Check sheet for the drawn part. Datum: minimum x, y, z corner. Units: mm. Coordinates: 2 decimals unless noted, no trailing zeros. Order: outer loops, then holes, each group sorted by start corner. A loop starts at its lowest first (then second) coordinate and runs counter-clockwise, first axis right, second up.
1. Cross-section at B-B (y = 23). Enter the section's corners in (x, z) (3 decimals).
2. Cross-section at A-A (z = 94). Enter the section's corners in (x, y) (3 decimals).
3. Gauge pin test, flat ends, axial feed: pin 1 Ø1.5 at (x, y) = (13, 133) entering from +Z; pin 2 Ø1.5 at (x, y) = (12, 131) entering from -Z; pin 3 Ø2.5 at (x, z) = (14, 68.5) entering from +Y. Record the tip position at first contact, or that the pin passes through.
4. Thickness scan on line 1 (Z direction, x = 14.75, y = 26); line 2 (X direction, y = 126, z = 55.5) (3 decimals); line 3 (Y direction, x = 15.25, z = 84.5). Record the ranges inside material, lowest first.
5. Cross-section at C-C (x = 6.35). Enter the section's corners in (y, z).
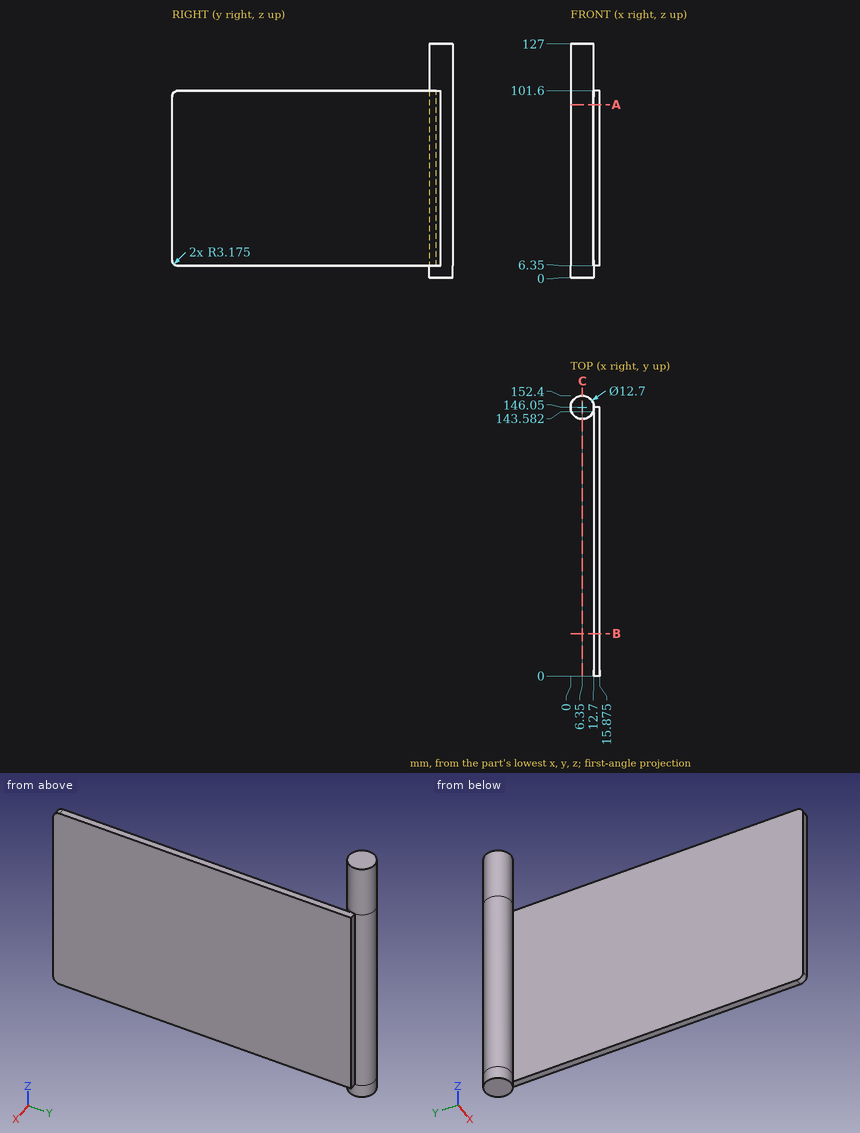
Data:
1. outline: (12.7, 6.35) - (15.875, 6.35) - (15.875, 101.6) - (12.7, 101.6) - close
2. outline: (12.201, 143.582) - (12.7, 143.582) - (12.7, 0) - (15.875, 0) - (15.875, 146.05) - (12.7, 146.05) arc R6.35 ccw (long way) to start
3. pin 1: stops at z = 101.6
3. pin 2: stops at z = 6.35
3. pin 3: stops at y = 146.05
4. line 1: z = 6.35 to 101.6
4. line 2: x = 12.7 to 15.875
4. line 3: y = 0 to 146.05
5. outline: (139.7, 0) - (152.4, 0) - (152.4, 127) - (139.7, 127) - close
